from build123d import *

# Parameters (mm, degrees)
F1_DEPTH = 28
F2_W     = 8
F2_H     = 10
F2_W_2   = 12.2721928373
F3_DEPTH = 25
F5_DEPTH = 25
F6_W     = 12
F6_H     = 10
F7_DEPTH = 25


with BuildPart() as f1:
    # F0 (on Top) → F1 (new body)
    with BuildSketch(Plane.XY):
        with BuildLine():
            ThreePointArc((-24.6996765713, -37.0061686144), (-16.2693027335, -40.9755360174), (-10.4808306919, -33.6734354945))
            ThreePointArc((-10.4808306919, -33.6734354945), (-10.7238019768, -31.7798848011), (-11.4369731527, -30.0090216931))
            Line((-11.4369731527, -30.0090216931), (-18.068324862, -33.5075951538))
            Line((-18.068324862, -33.5075951538), (-24.6996765713, -37.0061686144))
        make_face()
        with BuildLine():
            Line((-11.4369731527, -30.0090216931), (-50.5240537004, 39.792125391))
            ThreePointArc((-50.5240537004, 39.792125391), (-49.9919649413, 38.4837967792), (-49.81061565, 37.083098868))
            ThreePointArc((-49.81061565, 37.083098868), (-50.6007682567, 34.242792981), (-52.7441929341, 32.2185871305))
            Line((-52.7441929341, 32.2185871305), (-21.4804980317, -27.040010398))
            ThreePointArc((-21.4804980317, -27.040010398), (-15.8546767675, -26.4811153201), (-11.4369731527, -30.0090216931))
        make_face()
        with BuildLine():
            Line((-18.068324862, -33.5075951538), (-11.4369731527, -30.0090216931))
            ThreePointArc((-11.4369731527, -30.0090216931), (-15.8546767675, -26.4811153201), (-21.4804980317, -27.040010398))
            Line((-21.4804980317, -27.040010398), (-18.068324862, -33.5075951538))
        make_face()
        with BuildLine():
            Line((-60.2377675578, 34.639091078), (-24.6996765713, -37.0061686144))
            ThreePointArc((-24.6996765713, -37.0061686144), (-25.1177474282, -31.3681330201), (-21.4804980317, -27.040010398))
            Line((-21.4804980317, -27.040010398), (-52.7441929341, 32.2185871305))
            ThreePointArc((-52.7441929341, 32.2185871305), (-57.0011689379, 31.8493593272), (-60.2377675578, 34.639091078))
        make_face()
        with BuildLine():
            ThreePointArc((-21.4804980317, -27.040010398), (-25.1177474282, -31.3681330201), (-24.6996765713, -37.0061686144))
            Line((-24.6996765713, -37.0061686144), (-18.068324862, -33.5075951538))
            Line((-18.068324862, -33.5075951538), (-21.4804980317, -27.040010398))
        make_face()
        with BuildLine():
            ThreePointArc((-49.81061565, 37.083098868), (-49.9919649413, 38.4837967792), (-50.5240537004, 39.792125391))
            ThreePointArc((-50.5240537004, 39.792125391), (-57.8880915552, 41.9417630834), (-60.2377675578, 34.639091078))
            ThreePointArc((-60.2377675578, 34.639091078), (-57.0011689379, 31.8493593272), (-52.7441929341, 32.2185871305))
            ThreePointArc((-52.7441929341, 32.2185871305), (-50.6007682567, 34.242792981), (-49.81061565, 37.083098868))
        make_face()
    extrude(amount=F1_DEPTH)

    # F2 (on face) → F3 (cut)
    with BuildSketch(Plane(origin=(-34.5539816123, -17.1397598076, 0), x_dir=(0.4443650527, -0.8958458014, 0), z_dir=(-0.8958458014, -0.4443650527, 0))):
        with Locations((18.1761476979, 10)):
            Rectangle(F2_W, F2_H)
        with Locations((28.3122441165, 10)):
            Rectangle(F2_W_2, F2_H)
    extrude(amount=-F3_DEPTH, mode=Mode.SUBTRACT)

    # F4 (on face) → F5 (cut)
    with BuildSketch(Plane(origin=(-34.5539816123, -17.1397598076, 0), x_dir=(0.4443650527, -0.8958458014, 0), z_dir=(-0.8958458014, -0.4443650527, 0))):
        Polygon((-8.8238523021, 5), (11.1761476979, 5), (11.1761476979, 18), (-5.2653332241, 18), (-8.8238523021, 14.3358809873), align=None)
    extrude(amount=-F5_DEPTH, mode=Mode.SUBTRACT)

    # F6 (on face) → F7 (cut)
    with BuildSketch(Plane(origin=(-34.5539816123, -17.1397598076, 0), x_dir=(0.4443650527, -0.8958458014, 0), z_dir=(-0.8958458014, -0.4443650527, 0))):
        with Locations((-17.8238523021, 10)):
            Rectangle(F6_W, F6_H)
    extrude(amount=-F7_DEPTH, mode=Mode.SUBTRACT)


solid = f1.part
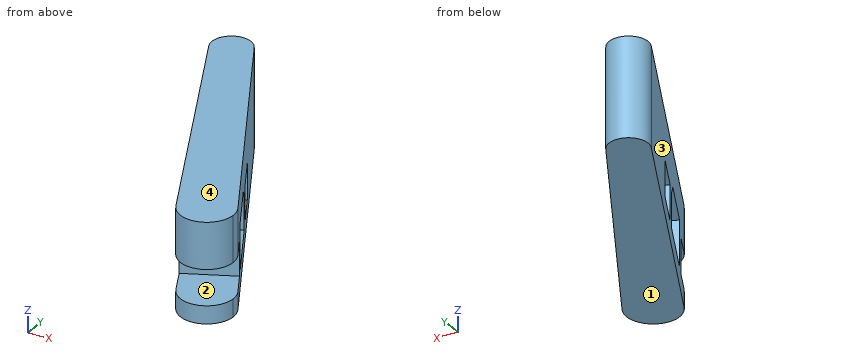
Check sheet for the modelled part. Datum: model origin and axes. Units: mm. Face numbers are marked on the shaded views. Round coordinates to 2 decimals unless told otherwise and drop trailing zeros. Write each loop counter-clockwise with the first axis right and the second up, starting at its lowest first coordinate (ties: lowest second). Pieces come first, ordered by that corner, then holes. Notation, with made-up numbers: (32, 7) -> (63, 7) arc R25 ccw to (63, 43) -> close; hole circle Ø5 at (46, 31.25). An arc over 180 degrees is marked (long way). Answer as CSV lines item,"result". Start each with the question number.
1) Section check A-A on z = 12.25. Enter the section's corners in (x, y) (1 decimal), and give its area (3 significant figures).
2) Material ranges on line 1 (Z direction, x = -43, y = 3); line 2 (Z direction, x = -31, y = -16); line 3 (Y direction, x = -28, z = 10.25), recorded low to high. Write a range as from..to.
3) Section check B-B on y = -32. Enter the section's corners in (x, z), and give its area (3 significant figures).
4) Release check for a two-part mould opening along Z. For the marked faces 1, 2, 3 and 4 record: pulls with the +Z half, pulls with the -Z half, needs draft (parallel to the pull), parting line crosses it, or undercut.
5) Section check C-C on z = 19. Enter the section's corners in (x, y).
6) Section check D-D on x = -20. Enter the section's corners in (y, z).
7) Go/stop test with flat-tipped pins: P1, Ø2, axis at y = -27, z = 11, coming from the +X side; P2, Ø8, axis at y = -3, z = 23.5, coming from the -X side; P3, Ø2, axis at x = -46, z = 17.5, coming from the +Y side. Record where each tip stops, or that it passes through.
Found:
1,outline,"(-60.2, 34.6) -> (-45.1, 4.2) -> (-33.8, 9.8) -> (-50.5, 39.7) arc R5.5 ccw to start; (-39.8, -6.5) -> (-38.5, -9.2) -> (-26.4, -3.3) -> (-27.9, -0.6) -> close; (-29.6, -27.2) -> (-28.3, -29.8) -> (-15.2, -23.3) -> (-16.6, -20.7) -> close"
1,area,"534 mm^2"
2,line 1,"z = 0..5, 15..28"
2,line 2,"z = 0..5, 18..28"
2,line 3,"y = -29.71..-26.36, -4.04..-0.69"
3,outline,"(-27.18, 0) -> (-10.67, 0) -> (-10.67, 5) -> (-27.18, 5) -> close; (-27.18, 15) -> (-10.67, 15) -> (-10.67, 28) -> (-27.18, 28) -> close"
3,area,"297 mm^2"
4,face 1,"pulls with the -Z half"
4,face 2,"undercut"
4,face 3,"needs draft"
4,face 4,"pulls with the +Z half"
5,outline,"(-60.24, 34.64) -> (-24.7, -37.01) arc R7.5 ccw (long way) to (-11.44, -30.01) -> (-50.5, 39.75) arc R5.5 ccw to start"
6,outline,"(-40.9, 0) -> (-14.72, 0) -> (-14.72, 5) -> (-22.4, 5) -> (-22.4, 18) -> (-14.72, 18) -> (-14.72, 28) -> (-40.9, 28) -> (-40.9, 15) -> (-25.74, 15) -> (-25.74, 5) -> (-40.9, 5) -> close"
7,P1,"stops at x = -20.51"
7,P2,"stops at x = -43.55"
7,P3,"stops at y = 33.5"
